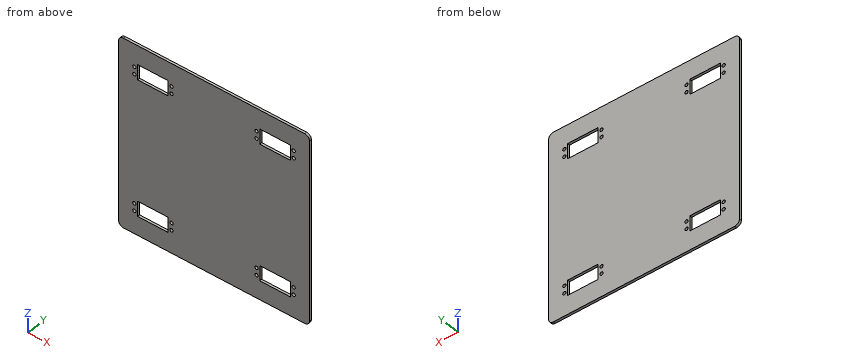
Autodesk Inventor part; units mm, degrees
ref_plane "YZ Plane" through (0, 0, 0) normal (1, 0, 0) x (0, 1, 0)
ref_plane "XZ Plane" through (0, 0, 0) normal (0, 1, 0) x (-1, 0, 0)
ref_plane "XY Plane" through (0, 0, 0) normal (0, 0, 1) x (1, 0, 0)
sketch "Sketch1" plane through (0, 0, 0) normal (0, 1, 0) x (-1, 0, 0)
  line L0 (0, 0) -> (-254, 0)
  line L1 (-254, 0) -> (-254, -254)
  line L2 (-254, -254) -> (0, -254)
  line L3 (0, -254) -> (0, 0)
  dimension "d0" = 254
  dimension "d1" = 254
extrude "Extrusion1" add sketch "Sketch1" along normal blind 3.175
fillet "Fillet1" radius 6.35 4 edges at (0, 1.5875, 0) (254, 1.5875, 0) (254, 1.5875, -254) (0, 1.5875, -254)
sketch "Sketch2" plane through (0, 3.175, 0) normal (0, 1, 0) x (1, 0, 0)
  line L0 (247.65, 254) -> (6.35, 254)
  line L1 (0, 247.65) -> (0, 6.35)
  line L2 (25.4, 45.72) -> (66.04, 45.72)
  line L3 (66.04, 45.72) -> (66.04, 25.4)
  line L4 (66.04, 25.4) -> (25.4, 25.4)
  line L5 (25.4, 25.4) -> (25.4, 45.72)
  line L6 (254, 6.35) -> (254, 247.65)
  line L7 (6.35, 0) -> (247.65, 0)
  circle A0 centre (20.955, 30.635) radius 2.1828
  circle A1 centre (20.955, 40.485) radius 2.1828
  circle A2 centre (70.485, 40.485) radius 2.1828
  circle A3 centre (70.485, 30.635) radius 2.1828
  line L8 (25.4, 228.6) -> (66.04, 228.6)
  line L9 (66.04, 228.6) -> (66.04, 208.28)
  line L10 (66.04, 208.28) -> (25.4, 208.28)
  line L11 (25.4, 208.28) -> (25.4, 228.6)
  circle A4 centre (20.955, 213.515) radius 2.1828
  circle A5 centre (20.955, 223.365) radius 2.1828
  circle A6 centre (70.485, 223.365) radius 2.1828
  circle A7 centre (70.485, 213.515) radius 2.1828
  circle A8 centre (233.045, 223.365) radius 2.1828
  circle A9 centre (233.045, 213.515) radius 2.1828
  line L12 (228.6, 228.6) -> (228.6, 208.28)
  line L13 (187.96, 228.6) -> (228.6, 228.6)
  line L14 (228.6, 208.28) -> (187.96, 208.28)
  line L15 (187.96, 208.28) -> (187.96, 228.6)
  circle A10 centre (183.515, 223.365) radius 2.1828
  circle A11 centre (183.515, 213.515) radius 2.1828
  circle A12 centre (233.045, 40.485) radius 2.1828
  circle A13 centre (233.045, 30.635) radius 2.1828
  line L16 (228.6, 45.72) -> (228.6, 25.4)
  line L17 (187.96, 45.72) -> (228.6, 45.72)
  line L18 (228.6, 25.4) -> (187.96, 25.4)
  line L19 (187.96, 25.4) -> (187.96, 45.72)
  circle A14 centre (183.515, 40.485) radius 2.1828
  circle A15 centre (183.515, 30.635) radius 2.1828
  point P0 (0, 0)
  point P1 (45.72, 25.4)
  point P2 (25.4, 35.56)
  point P3 (45.72, 208.28)
  point P4 (25.4, 218.44)
  point P5 (127, 254)
  point P6 (208.28, 208.28)
  point P7 (187.96, 218.44)
  point P8 (208.28, 25.4)
  point P9 (187.96, 35.56)
  point P10 (208.28, 228.6)
  dimension "d13" = 40.64
  dimension "d14" = 20.32
  dimension "d19" = 25.4
  dimension "d20" = 25.4
  dimension "d23" = 4.3656
  dimension "d24" = 4.3656
  dimension "d25" = 4.3656
  dimension "d26" = 4.3656
  dimension "d27" = 9.85
  dimension "d28" = 9.85
  dimension "d29" = 49.53
  dimension "d30" = 49.53
  dimension "d31" = 0
  dimension "d32" = 0
  dimension "d33" = 4.445
  dimension "d34" = 5.235
  dimension "d35" = 40.64
  dimension "d36" = 20.32
  dimension "d37" = 4.3656
  dimension "d38" = 4.3656
  dimension "d39" = 4.3656
  dimension "d40" = 4.3656
  dimension "d41" = 9.85
  dimension "d42" = 9.85
  dimension "d43" = 49.53
  dimension "d44" = 49.53
  dimension "d45" = 0
  dimension "d46" = 0
  dimension "d47" = 4.445
  dimension "d48" = 5.235
  dimension "d51" = 25.4
  dimension "d52" = 25.4
  dimension "d53" = 40.64
  dimension "d54" = 20.32
  dimension "d55" = 4.3656
  dimension "d56" = 4.3656
  dimension "d57" = 4.3656
  dimension "d58" = 4.3656
  dimension "d59" = 9.85
  dimension "d60" = 9.85
  dimension "d61" = 49.53
  dimension "d62" = 49.53
  dimension "d63" = 0
  dimension "d64" = 0
  dimension "d65" = 4.445
  dimension "d66" = 5.235
  dimension "d69" = 40.64
  dimension "d70" = 20.32
  dimension "d71" = 4.3656
  dimension "d72" = 4.3656
  dimension "d73" = 4.3656
  dimension "d74" = 4.3656
  dimension "d75" = 9.85
  dimension "d76" = 9.85
  dimension "d77" = 49.53
  dimension "d78" = 49.53
  dimension "d79" = 0
  dimension "d80" = 0
  dimension "d81" = 4.445
  dimension "d82" = 5.235
  dimension "d85" = 25.4
  dimension "d86" = 25.4
  dimension "d87" = 25.4
  dimension "d88" = 25.4
extrude "Extrusion2" cut sketch "Sketch2" against normal blind 3.175
equation "\"d13\" = d5"
equation "\"d14\" = d6"
equation "\"d28\" = d27"
equation "\"d29\" = d30"
equation "\"d33\" = -0.5 * d13 + 0.5 * d29"
equation "\"d34\" = -0.5 * d27 + 0.5 * d14"
equation "\"d35\" = d49"
equation "\"d36\" = d50"
equation "\"d42\" = d41"
equation "\"d43\" = d44"
equation "\"d47\" = -0.5 * d35 + 0.5 * d43"
equation "\"d48\" = -0.5 * d41 + 0.5 * d36"
equation "\"d53\" = d67"
equation "\"d54\" = d68"
equation "\"d60\" = d59"
equation "\"d61\" = d62"
equation "\"d65\" = -0.5 * d53 + 0.5 * d61"
equation "\"d66\" = -0.5 * d59 + 0.5 * d54"
equation "\"d69\" = d83"
equation "\"d70\" = d84"
equation "\"d76\" = d75"
equation "\"d77\" = d78"
equation "\"d81\" = -0.5 * d69 + 0.5 * d77"
equation "\"d82\" = -0.5 * d75 + 0.5 * d70"
properties part number "RobotBase" material "Bronze, Cast"
Work out the finished part from the listing and answer in its coordinate system (mm). Coordinates: 2 decimals unless noted, no trailing zeros. Write each loop counter-clockwise with the first axis right and the second up, starting at its lowest first coordinate (ties: lowest second). Pieces come first, ordered by that corner, then holes. Notation, with made-up numbers: (28.25, -5.75) - (75.25, -5.75) arc R23 ccw to (75.25, 2.25) - close; hole circle Ø10 at (85, -28). An arc over 180 degrees is marked (long way). Answer as a JSON object with one key per item and string values.
Q1. Given pin 1 Ø3.5 at (x, z) = (183.515, -223.365) entering from +Y, flat-ended and moving along its own axis, determine where the tip first touches the part or whether it passes through.
Results list:
{"pin 1": "passes through"}
Q2. Find section A-A (x = 37). Write down the section's boundary in (y, z) (3 decimals).
Results list:
{"outline": "(0, -254) - (3.175, -254) - (3.175, -228.6) - (0, -228.6) - close; (0, -208.28) - (3.175, -208.28) - (3.175, -45.72) - (0, -45.72) - close; (0, -25.4) - (3.175, -25.4) - (3.175, 0) - (0, 0) - close"}
Q3. Find section B-B (y = 1.2). State how many separate pieces and enclosed holes the cut face has, plus the area to 3 significant figures.
Results list:
{"separate pieces": "1", "enclosed holes": "20", "area": "60,900 mm^2"}
Q4. Consider L1, parallel to Z at x = 199.5, y = 0.4; L2, parallel to X at y = 2.65, z = -37.5; L3, parallel to Z at x = 182.5, y = 2.45. Determine where each line is inside the solid, lowest interval first. Write a range as from..to.
Results list:
{"L1": "z = -254..-228.6, -208.28..-45.72, -25.4..0", "L2": "x = 0..25.4, 66.04..187.96, 228.6..254", "L3": "z = -254..-225.3, -221.43..-215.45, -211.58..-42.42, -38.55..-32.57, -28.7..0"}
